Can you work these out from the drawing? Everything is in mm from the part's minimum corner. Round coordinates to 2 decimals unless told otherwise and drop trailing zeros. Loops run counter-clockwise (first coordinate to the right, second up) from the corner with the lowest first, then second, coordinate; pieces in that order, holes last. Notation, with made-up numbers: M 41.25,61 L 86.25,61 A12 cw 86.25,67 Z; hole C -33,-5.5 d4. An arc over 180 degrees is marked long. Return JSON: item names as keys, results as strings. Group by question number.
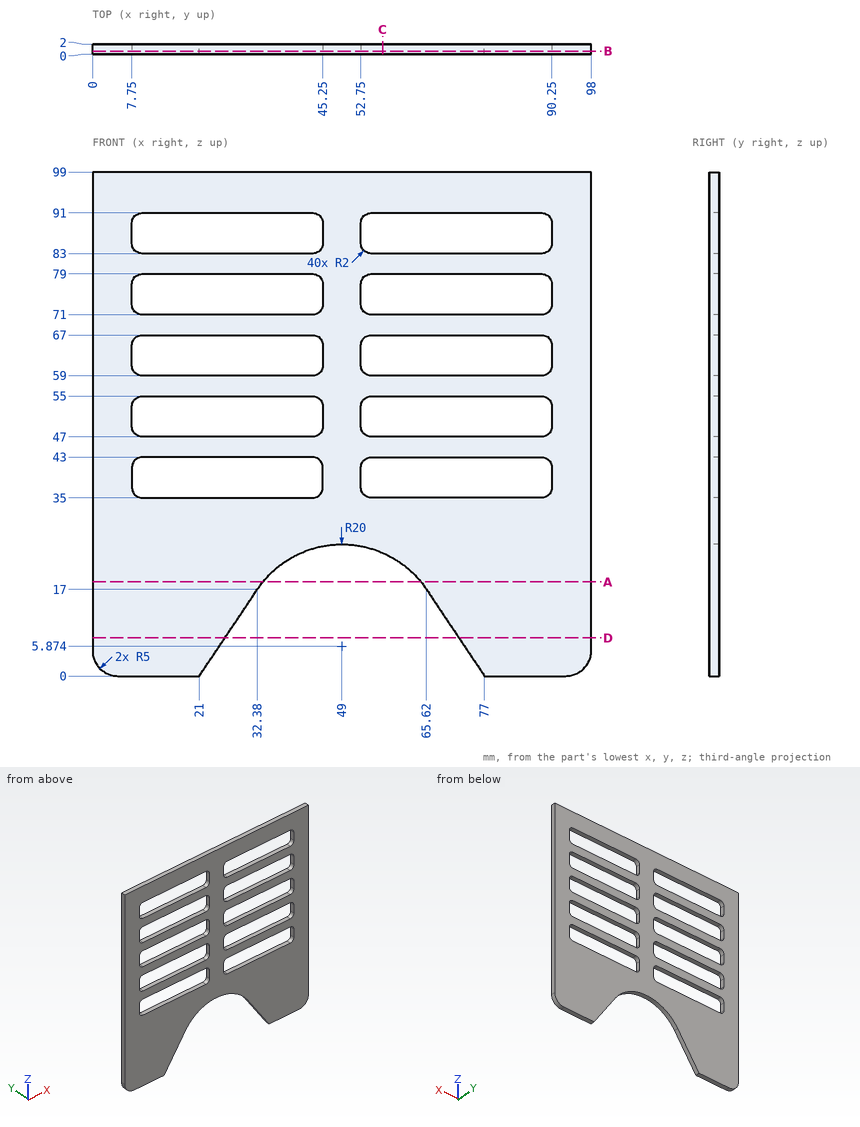
1. I need wall thicknesses on probe 1 along Z at (x, y) = (81, 1.45); probe 2 along X at (y, z) = (0.45, 39); probe 3 along Z at (x, y) = (89.5, 0.9). Which ranges of each line are inside material? Lowest first, please.
2. If we section it at C-C, the plane x = 57: Please give me the cut outline in (y, z) (1 decimal).
3. If we section it at B-B, the plane y = 0.6: Give the number of separate pieces and of enclosed holes in the cut face, then the cut area to 3 significant figures.
4. If we section it at D-D, the plane z = 7.5: Please give me the cut outline in (x, y), then the cut area to 3 significant figures.
5. I'm going to push flat-ended pins straight in: pin 1 Ø0.6 at (x, y) = (74.5, 1) entering from -Z (1 decimal); pin 2 Ø0.6 at (x, y) = (67, 0.5) entering from -Z. Where does each tip first touch, or does it pass through?
6. If we section it at A-A, the plane z = 18.5: Please give me the cut outline in (x, y), then the cut area to 3 significant figures.
Geometry results:
{
 "1": {"probe 1": "0 to 35, 43 to 47, 55 to 59, 67 to 71, 79 to 83, 91 to 99", "probe 2": "0 to 7.75, 45.25 to 52.75, 90.25 to 98", "probe 3": "0 to 35.44, 42.56 to 47.44, 54.56 to 59.44, 66.56 to 71.44, 78.56 to 83.44, 90.56 to 99"},
 "2": {"outline": "M 0,24.2 L 2,24.2 L 2,35 L 0,35 Z; M 0,43 L 2,43 L 2,47 L 0,47 Z; M 0,55 L 2,55 L 2,59 L 0,59 Z; M 0,67 L 2,67 L 2,71 L 0,71 Z; M 0,79 L 2,79 L 2,83 L 0,83 Z; M 0,91 L 2,91 L 2,99 L 0,99 Z"},
 "3": {"separate pieces": "1", "enclosed holes": "10", "area": "5,760 mm^2"},
 "4": {"outline": "M 0,0 L 26.02,0 L 26.02,2 L 0,2 Z; M 71.98,0 L 98,0 L 98,2 L 71.98,2 Z", "area": "104 mm^2"},
 "5": {"pin 1": "z = 3.3", "pin 2": "z = 14.49"},
 "6": {"outline": "M 0,0 L 33.49,0 L 33.49,2 L 0,2 Z; M 64.51,0 L 98,0 L 98,2 L 64.51,2 Z", "area": "134 mm^2"}
}
